Read the model definition and answer for the solid it produces. Units are mm, in the model's axes. Coordinates: 2 decimals unless noted, no trailing zeros. Write each loop counter-clockwise with the first axis right and the second up, starting at its lowest first coordinate (ties: lowest second). Pieces come first, ordered by that corner, then holes.
(1) Given pin 1 (5 mm diameter, centred on x = 75.5, z = -75.5, fed in from +Y), flat-ended and moving along its own axis, determine where the tip first touches the part or whether it passes through.
(2) The mould has two halves that part along X. Classify faces 1 (the cylindrical face through (74, 3, -59)), 2 (the cylindrical face through (121.99, 3.22, -87.15)), 3 (the cylindrical face through (2.85, 3.22, -86.99)), 4 (the cylindrical face through (56.086, 3.219, -57.161)): +X half, -X half, draft (parallel to the pull), parting line (faces both ways), or undercut.
(3) Section A-A on x = 107 is taken. Write down the section's boundary in (y, z).
(4) Section D-D on z = -51 is taken. Write down the section's boundary in (x, y).
(5) Find the intervals of material crossed by probe 1 along X at (y, z) = (2, -29.5); probe 2 along Z at (x, y) = (108, 1.75); probe 3 along Z at (x, y) = (92, 5.5), in increasing order.
(6) Section C-C on x = 91.5 is taken. Write down the section's boundary in (y, z), then the cut area to 3 significant figures.
(7) Section B-B on z = -75.5 is taken. Write down the section's boundary in (x, y).
from build123d import *

# Parameters (mm, degrees)
BOSS_EXTRUDE1_OUTLINE_W = 125
BOSS_EXTRUDE1_OUTLINE_H = 90
BOSS_EXTRUDE1_DEPTH     = 6.35
SKETCH2_R               = 3
CUT_EXTRUDE1_DEPTH      = 10
SKETCH3_R               = 4.5
SKETCH3_R_2             = 2.5
SERVO_CUTOUT_DEPTH      = 10
FILLET1_R               = 10
SKETCH4_R               = 15.825603453
CUT_EXTRUDE3_DEPTH      = 10


# Read off the part's stored shape, not the designer's step: Boss-Extrude1
with BuildPart() as part:
    # Boss-Extrude1 outline → Boss-Extrude1 (new body)
    with BuildSketch(Plane(origin=(0, 0, 0), x_dir=(1, 0, 0), z_dir=(0, 1, 0))):
        with Locations((62.5, 45)):
            Rectangle(BOSS_EXTRUDE1_OUTLINE_W, BOSS_EXTRUDE1_OUTLINE_H)
    extrude(amount=BOSS_EXTRUDE1_DEPTH)

    # Sketch2 → Cut-Extrude1 (cut)
    with BuildSketch(Plane(origin=(0, 6.35, 0), x_dir=(1, 0, 0), z_dir=(0, 1, 0))):
        with Locations(Location((14.5, 14.5, 0), (0, 0, 270))):
            Circle(SKETCH2_R)
        with Locations(Location((75.5, 14.5, 0), (0, 0, 270))):
            Circle(SKETCH2_R)
        with Locations(Location((75.5, 75.5, 0), (0, 0, 270))):
            Circle(SKETCH2_R)
        with Locations(Location((14.5, 75.5, 0), (0, 0, 270))):
            Circle(SKETCH2_R)
    extrude(amount=-CUT_EXTRUDE1_DEPTH, mode=Mode.SUBTRACT)

    # Sketch3 → Servo_Cutout (cut)
    with BuildSketch(Plane(origin=(0, 6.35, 0), x_dir=(1, 0, 0), z_dir=(0, 1, 0))):
        with Locations(Location((91.5, 45, 0), (0, 0, 270))):
            Circle(SKETCH3_R)
        with Locations(Location((107, 60.5, 0), (0, 0, 270))):
            Circle(SKETCH3_R_2)
        with Locations(Location((76, 60.5, 0), (0, 0, 270))):
            Circle(SKETCH3_R_2)
        with Locations(Location((76, 29.5, 0), (0, 0, 270))):
            Circle(SKETCH3_R_2)
        with Locations(Location((107, 29.5, 0), (0, 0, 270))):
            Circle(SKETCH3_R_2)
    extrude(amount=-SERVO_CUTOUT_DEPTH, mode=Mode.SUBTRACT)

    # Fillet1
    fillet1_edges = [part.edges().sort_by_distance(p)[0] for p in [
        (0, 3.175, -90),
        (125, 3.175, -90),
        (125, 3.175, 0),
        (0, 3.175, 0),
    ]]
    fillet(fillet1_edges, radius=FILLET1_R)

    # Sketch4 → Cut-Extrude3 (cut)
    with BuildSketch(Plane(origin=(0, 6.35, 0), x_dir=(1, 0, 0), z_dir=(0, 1, 0))):
        with Locations(Location((45.38988598, 45.496671395, 0), (0, 0, 270))):
            Circle(SKETCH4_R)
    extrude(amount=-CUT_EXTRUDE3_DEPTH, mode=Mode.SUBTRACT)


solid = part.part
Response:
1. pin 1: passes through
2. face 1: undercut
2. face 2: +X half
2. face 3: -X half
2. face 4: undercut
3. outline: (0, -90) - (6.35, -90) - (6.35, -63) - (0, -63) - close; (0, -58) - (6.35, -58) - (6.35, -32) - (0, -32) - close; (0, -27) - (6.35, -27) - (6.35, 0) - (0, 0) - close
4. outline: (0, 0) - (30.55, 0) - (30.55, 6.35) - (0, 6.35) - close; (60.23, 0) - (125, 0) - (125, 6.35) - (60.23, 6.35) - close
5. probe 1: x = 0 to 73.5, 78.5 to 104.5, 109.5 to 125
5. probe 2: z = -90 to -62.79, -58.21 to -31.79, -27.21 to 0
5. probe 3: z = -90 to -49.47, -40.53 to 0
6. outline: (0, -90) - (6.35, -90) - (6.35, -49.5) - (0, -49.5) - close; (0, -40.5) - (6.35, -40.5) - (6.35, 0) - (0, 0) - close
6. area: 514 mm2
7. outline: (0, 0) - (11.5, 0) - (11.5, 6.35) - (0, 6.35) - close; (17.5, 0) - (72.5, 0) - (72.5, 6.35) - (17.5, 6.35) - close; (78.5, 0) - (125, 0) - (125, 6.35) - (78.5, 6.35) - close
